Geometry: final body of the model. Coordinates: model frame, mm. A direction names the side the tool comes from. Round coordinates to 2 decimals unless told otherwise and drop trailing zeros. Write each loop counter-clockwise with the first axis right and the second up, starting at its lowest first coordinate (ties: lowest second). Pieces come first, ordered by that corner, then holes. Notation, with made-up numbers: (47.25, -40) - (68.25, -40) arc R28 cw to (68.25, -9) - close; hole circle Ø6 at (-33, 41). An arc over 180 degrees is marked (long way). Use a Markdown table: item, result. Add a question column.
```python
from build123d import *

# Parameters (mm, degrees)
F1_DEPTH  = 200
F2_R      = 199.99999
F3_R      = 125
F4_DEPTH  = 50
F5_R      = 125
F6_DEPTH  = 50
F7_R      = 75
F8_DEPTH  = 350
F9_R      = 75
F10_DEPTH = 312.5


# Not quite as in the source:
# - a fillet or chamfer is up to 0.001 mm smaller than in the source, because OpenCascade refuses the exact size
# - a pattern or mirror of a feature is missing from the dataset's text; its kind, count and spacing are read off the source's solid


with BuildPart() as f1:
    # F0 (on Front) → F1 (new body, symmetric)
    with BuildSketch(Plane.XZ):
        with BuildLine():
            ThreePointArc((250, 150), (220.7106781187, 220.7106781187), (150, 250))
            Line((150, 250), (-150, 250))
            ThreePointArc((-150, 250), (-220.7106781187, 220.7106781187), (-250, 150))
            Line((-250, 150), (-250, -250))
            Line((-250, -250), (-150, -250))
            Line((-150, -250), (-150, 50))
            ThreePointArc((-150, 50), (-120.7106781187, 120.7106781187), (-50, 150))
            Line((-50, 150), (50, 150))
            ThreePointArc((50, 150), (120.7106781187, 120.7106781187), (150, 50))
            Line((150, 50), (150, -250))
            Line((150, -250), (250, -250))
            Line((250, -250), (250, 150))
        make_face()
    extrude(amount=F1_DEPTH, both=True)

    # F2 (radius 200 in the source; OpenCascade refuses exactly that, so slightly less here)
    f2_edges = [f1.edges().sort_by_distance(p)[0] for p in [
        (-200, -200, -250),
        (-200, 200, -250),
        (200, -200, -250),
        (200, 200, -250),
    ]]
    fillet(f2_edges, radius=F2_R)

    # F3 (on face) → F4 (join)
    with BuildSketch(Plane.YZ.offset(250)):
        with Locations((0, -50)):
            Circle(F3_R)
    f4 = extrude(amount=F4_DEPTH)

    # F4_copies: F4 across plane
    add(f4.mirror(Plane(origin=(0, 0, 0), x_dir=(0, 0, -1), z_dir=(-1, 0, 0))))

    # F5 (on face) → F6 (join)
    with BuildSketch(Plane.XY.offset(250)):
        Circle(F5_R)
    extrude(amount=F6_DEPTH)

    # F7 (on Right) → F8 (cut, symmetric)
    with BuildSketch(Plane.YZ):
        with Locations((0, -50)):
            Circle(F7_R)
    extrude(amount=F8_DEPTH, both=True, mode=Mode.SUBTRACT)

    # F9 (on face) → F10 (cut)
    with BuildSketch(Plane.XY.offset(300)):
        Circle(F9_R)
    extrude(amount=-F10_DEPTH, mode=Mode.SUBTRACT)


solid = f1.part
```
1) Material intervals for L1, parallel to X at y = -14.5, z = -169; L2, parallel to X at y = 122.5, z = -169.5; L3, parallel to Z at x = -257, y = 0, sorted ascending. Write a range as from..to.
2) Draft query along X for faces 6 (the flat face through (54, -54, 300)), 7 (the flat face through (-300, 54, -104)), 8 (the flat face through (300, 54, -104)), 9 (the cylindrical face through (-121.484, -2.8, 119.929)). Return one class per face: released by +X, released by -X, zero draft, split by the parting line, or undercut.
3) Set-up query: faces 1 (the cylindrical face through (-223.95, -16.259, -123.217)), 2 (the flat face through (2, -136, 250)), 3 (the flat face through (-1, 127, 150)), 4 (the cylindrical face through (274.65, -124.88, -44.5)), 5 (the cylindrical face through (-274.65, -124.88, -44.5)). Return all of +Z, -Z, +X, -X, +Y, -Y with unobstructed straight access to the full face (end or side cutting, diameter ignored); none if empty.
4) Section B-B, the plane z = -82. Return the cut outline in (x, y), then the cut area to 3 significant figures.
5) Section D-D, the plane y = 102.5. Return the cut outline in (x, z).
6) Section A-A, the plane x = 0. Return the cut outline in (y, z).
7) Pin query (flat end, axial travel): P1, Ø5, axis at y = -125.5, z = 161.5, coming from the -X side; P2, Ø1, axis at x = -219, y = -146, coming from the +Z side; P3, Ø1, axis at y = 37.5, z = 118, coming from the +X side. Return the tip coordinate at first contact, or that it passes through.
Output values:
| question | item | result |
|---|---|---|
| 1 | L1 | x = -300..-150, 150..300 |
| 1 | L2 | x = -250..-150, 150..250 |
| 1 | L3 | z = -175..-125, 25..75 |
| 2 | face 6 | zero draft |
| 2 | face 7 | released by -X |
| 2 | face 8 | released by +X |
| 2 | face 9 | undercut |
| 3 | face 1 | +X, -X |
| 3 | face 2 | +Z |
| 3 | face 3 | -Z, +Y, -Y |
| 3 | face 4 | +X |
| 3 | face 5 | -X |
| 4 | outline | (-300, -120.83) - (-250, -120.83) - (-250, -197.42) - (-150, -197.42) - (-150, -67.83) - (-300, -67.83) - close; (-300, 67.83) - (-150, 67.83) - (-150, 197.42) - (-250, 197.42) - (-250, 120.83) - (-300, 120.83) - close; (150, -197.42) - (250, -197.42) - (250, -120.83) - (300, -120.83) - (300, -67.83) - (150, -67.83) - close; (150, 67.83) - (300, 67.83) - (300, 120.83) - (250, 120.83) - (250, 197.42) - (150, 197.42) - close |
| 4 | area | 62,400 mm^2 |
| 5 | outline | (-300, -121.55) - (-250, -121.55) - (-250, -221.74) - (-150, -221.74) - (-150, 50) arc R100 cw to (-50, 150) - (50, 150) arc R100 cw to (150, 50) - (150, -221.74) - (250, -221.74) - (250, -121.55) - (300, -121.55) - (300, 21.55) - (250, 21.55) - (250, 150) arc R100 ccw to (150, 250) - (71.55, 250) - (71.55, 300) - (-71.55, 300) - (-71.55, 250) - (-150, 250) arc R100 ccw to (-250, 150) - (-250, 21.55) - (-300, 21.55) - close |
| 6 | outline | (-200, 150) - (-75, 150) - (-75, 300) - (-125, 300) - (-125, 250) - (-200, 250) - close; (75, 150) - (200, 150) - (200, 250) - (125, 250) - (125, 300) - (75, 300) - close |
| 7 | P1 | stops at x = -249.59 |
| 7 | P2 | stops at z = 222.85 |
| 7 | P3 | stops at x = 250 |
